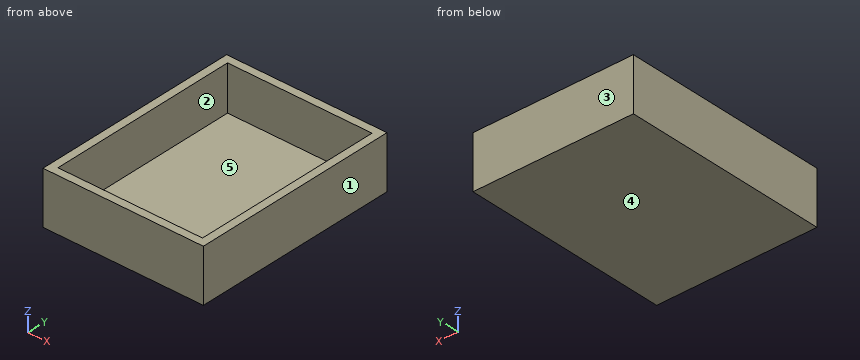
from build123d import *

# Parameters (mm, degrees)
F0_W     = 364
F0_H     = 470
F1_DEPTH = 60
F2_W     = 328
F2_H     = 434
F3_DEPTH = 102


with BuildPart() as f1:
    # F0 (on Top) → F1 (new body, symmetric)
    with BuildSketch(Plane.XY):
        Rectangle(F0_W, F0_H)
    extrude(amount=F1_DEPTH, both=True)

    # F2 (on face) → F3 (cut)
    with BuildSketch(Plane.XY.offset(60)):
        Rectangle(F2_W, F2_H)
    extrude(amount=-F3_DEPTH, mode=Mode.SUBTRACT)


solid = f1.part
The model under review builds one solid part; all positions refer to its coordinate system, in mm. Face numbers are marked on the shaded views. A direction names the side the tool comes from. Round coordinates to 2 decimals unless told otherwise and drop trailing zeros. Loops run counter-clockwise (first coordinate to the right, second up) from the corner with the lowest first, then second, coordinate; pieces in that order, holes last. Notation, with made-up numbers: (-34.5, 53.25) -> (8.5, 53.25) arc R27 cw to (8.5, 74.25) -> close; hole circle Ø7 at (55.25, 44). An arc over 180 degrees is marked (long way). One line per question, with ' | ' between items. Start each with the question number.
Item 1: Add section B-B, the plane y = 80.5. Write out the cut boundary in (x, z).
Item 2: Add section C-C, the plane x = -71. Write out the cut boundary in (y, z), then the cut area to 3 significant figures.
Item 3: Wall thickness on line 1 along X through (y, z) = (-39.5, 24); line 2 along Y through (x, z) = (34, -20); line 3 along Z through (x, y) = (24, -50.5): over which ranges is each line inside the solid? List them lowest first. Write a range as [from, to].
Item 4: Add section A-A, the plane z = -14.5. Write out the cut boundary in (x, y).
Item 5: Machinability: for the marked faces 4 and 5, which of the approach directions +Z, -Z, +X, -X, +Y, -Y give a long, thin tool a straight path to every point of the face, cutting with its end or side? Answer none if there is none.
Item 6: Draft analysis for pull direction Y (two halves, no side actions). For the marked faces 1, 2 and 3, state which applies: +Y half, -Y half, draft (parallel to the pull), parting line (faces both ways), or undercut.
Return value:
1) outline: (-182, -60) -> (182, -60) -> (182, 60) -> (164, 60) -> (164, -42) -> (-164, -42) -> (-164, 60) -> (-182, 60) -> close
2) outline: (-235, -60) -> (235, -60) -> (235, 60) -> (217, 60) -> (217, -42) -> (-217, -42) -> (-217, 60) -> (-235, 60) -> close | area: 12,100 mm2
3) line 1: x = [-182, -164], [164, 182] | line 2: y = [-235, -217], [217, 235] | line 3: z = [-60, -42]
4) outline: (-182, -235) -> (182, -235) -> (182, 235) -> (-182, 235) -> close; hole (-164, -217) -> (164, -217) -> (164, 217) -> (-164, 217) -> close
5) face 4: -Z, +X, -X, +Y, -Y | face 5: +Z
6) face 1: draft | face 2: undercut | face 3: +Y half
